For this review, use the dimensioned drawing (mm, ordinates from the lowest corner) and the shaded views. A direction names the side the tool comes from. Coordinates: 2 decimals unless noted, no trailing zeros. Loops run counter-clockwise (first coordinate to the right, second up) from the corner with the lowest first, then second, coordinate; pieces in that order, holes last. Notation, with made-up numbers: (-22.5, -12) - (6.5, -12) arc R26 ccw to (6.5, 8) - close; hole circle Ø3 at (-1.75, -19.5). An arc over 180 degrees is marked (long way). Use a Markdown table: item, result. Add a question column.
1) The part is to be moulded in two halves that separate along Y. For the marked faces 1, 2 and 3, say which applies: pulls with the +Y half, pulls with the -Y half, needs draft (parallel to the pull), parting line crosses it, or undercut.
2) Add section B-B, the plane x = 51.5. Give the boundary of the cut face in (y, z), and give its area (3 significant figures).
3) To check wall thickness, follow L1, parallel to Y at x = 15, z = 41.8; L2, parallel to Y at x = 46, z = 44.5. State the ranges of each line that lie inside material, in increasing order. Write a range as [from, to].
4) Add section A-A, the plane z = 45. Give the boundary of the cut face in (x, y), and give its area (3 significant figures).
5) For the marked faces 4 and 5, list the 3-axis set-ups (+Z, -Z, +X, -X, +Y, -Y) from which the entire face can be reached by the end or side of a thin tool; tool diameter is ignored.
6) Add section D-D, the plane z = 16.5. Give the number of separate pieces and of enclosed holes in the cut face, and give its area (3 significant figures).
7) Clearance check with flat-ended pins moving along their axes: pin 1 (1 mm diameter, centred on x = 26.5, y = 40.5, fed in from -Z); pin 2 (3 mm diameter, centred on x = 20.5, y = 41, fed in from +Z). State where each tip first meets the part, or that it passes through.
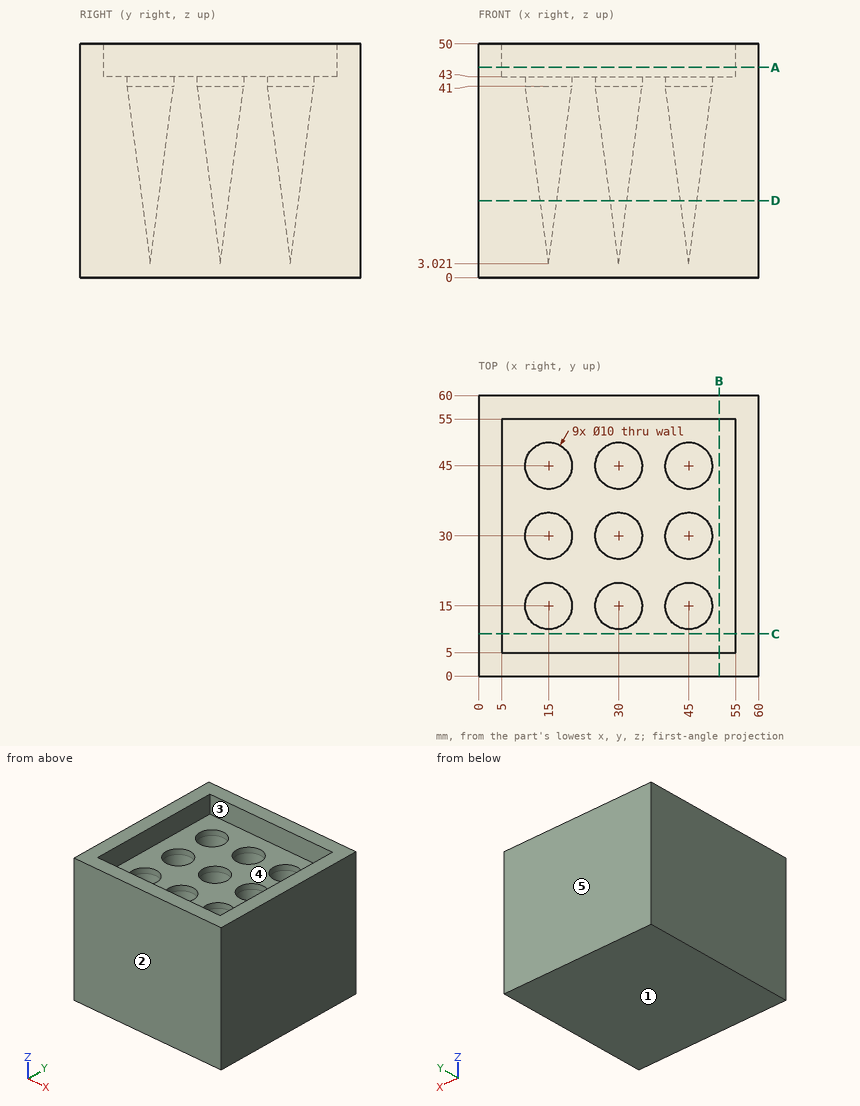
From the geometry:
| question | item | result |
|---|---|---|
| 1 | face 1 | needs draft |
| 1 | face 2 | pulls with the -Y half |
| 1 | face 3 | undercut |
| 2 | outline | (0, 0) - (60, 0) - (60, 50) - (55, 50) - (55, 43) - (5, 43) - (5, 50) - (0, 50) - close |
| 2 | area | 2,650 mm^2 |
| 3 | L1 | y = [0, 10], [20, 25], [35, 40], [50, 60] |
| 3 | L2 | y = [0, 5], [55, 60] |
| 4 | outline | (0, 0) - (60, 0) - (60, 60) - (0, 60) - close; hole (5, 5) - (55, 5) - (55, 55) - (5, 55) - close |
| 4 | area | 1,100 mm^2 |
| 5 | face 4 | +Z |
| 5 | face 5 | +Z, -Z, +X, -X, +Y |
| 6 | separate pieces | 1 |
| 6 | enclosed holes | 9 |
| 6 | area | 3,510 mm^2 |
| 7 | pin 1 | stops at z = 0 |
| 7 | pin 2 | stops at z = 43 |
